```python
from build123d import *

# Parameters (mm, degrees)
BOSS_EXTRU_1_DEPTH       = 35
COQUE3_T                 = 2
ESQUISSE3_R              = 13
ENL_V_MAT_EXTRU_1_DEPTH  = 82.443231763
ESQUISSE5_W              = 20
ESQUISSE5_H              = 5
ENL_V_MAT_EXTRU_3_DEPTH  = 2
ESQUISSE6_R              = 4.6
ENL_V_MAT_EXTRU_4_DEPTH  = 122.428991596
ESQUISSE7_R              = 2.1
ENL_V_MAT_EXTRU_5_DEPTH  = 122.428991596
ESQUISSE8_W              = 44
ESQUISSE8_H              = 20
BOSS_EXTRU_2_DEPTH       = 17
ESQUISSE9_W              = 40
ESQUISSE9_H              = 15
ENL_V_MAT_EXTRU_7_DEPTH  = 18
ESQUISSE10_W             = 3
ESQUISSE10_H             = 6
ENL_V_MAT_EXTRU_8_DEPTH  = 5
BOSS_EXTRU_4_DEPTH       = 3
ESQUISSE22_R             = 4.5
BOSS_EXTRU_7_DEPTH       = 1
ENL_V_START              = -3
ESQUISSE24_R             = 2.1
ENL_V_MAT_EXTRU_12_DEPTH = 3
ESQUISSE20_R             = 4.5
BOSS_EXTRU_8_DEPTH       = 1
ESQUISSE25_R             = 2.1
ENL_V_MAT_EXTRU_13_DEPTH = 3
BOSS_EXTRU_9_START       = 1
ESQUISSE26_R             = 4.5
BOSS_EXTRU_9_DEPTH       = 1
ESQUISSE27_R             = 2.1
ENL_V_MAT_EXTRU_14_DEPTH = 3
BOSS_EXTRU_10_START      = 1
ESQUISSE28_R             = 4.5
BOSS_EXTRU_10_DEPTH      = 1
ESQUISSE29_R             = 2.1
ENL_V_MAT_EXTRU_15_DEPTH = 3
ESQUISSE34_R             = 5.75
BOSS_EXTRU_16_DEPTH      = 1
ESQUISSE35_R             = 4.6
ENL_V_MAT_EXTRU_19_DEPTH = 1
ESQUISSE36_R             = 5.5
BOSS_EXTRU_17_DEPTH      = 1
ESQUISSE37_R             = 4.6
ENL_V_MAT_EXTRU_20_DEPTH = 1
NERVURE3_REACH           = 96.86
ESQUISSE38_WALL_W        = 204.379203954
ESQUISSE38_WALL_H        = 2
NERVURE4_REACH           = 120.87
ESQUISSE39_WALLS_W       = 252.639353074
ESQUISSE39_WALLS_H       = 2
ESQUISSE40_W             = 24
ESQUISSE40_H             = 20
ENL_V_MAT_EXTRU_21_DEPTH = 2
SYM_TRIE2_START          = 12.2
SYM_TRIE2_OUTLINE_W      = 1
SYM_TRIE2_OUTLINE_H      = 11.067979308
SYM_TRIE2_DEPTH          = 2


with BuildPart() as part:
    # Esquisse1 → Boss.-Extru.1 (new body)
    with BuildSketch(Plane.XY):
        Polygon((-50, 20), (-20, 50), (20, 50), (50, 20), (50, -50), (-50, -50), align=None)
    extrude(amount=BOSS_EXTRU_1_DEPTH)

    # Coque3
    coque3_openings = [part.faces().sort_by_distance(p)[0] for p in [
        (0, -3.956043956, 35),
    ]]
    offset(amount=COQUE3_T, openings=coque3_openings, kind=Kind.INTERSECTION)

    # Esquisse3 → Enlèv. mat.-Extru.1 (cut, through all)
    with BuildSketch(Plane.XY):
        Circle(ESQUISSE3_R)
    extrude(amount=-ENL_V_MAT_EXTRU_1_DEPTH, mode=Mode.SUBTRACT)

    # Esquisse5 → Enlèv. mat.-Extru.3 (cut)
    with BuildSketch(Plane.XZ.offset(52)):
        with Locations((39, 3.5)):
            Rectangle(ESQUISSE5_W, ESQUISSE5_H)
        with Locations((-39, 3.5)):
            Rectangle(ESQUISSE5_W, ESQUISSE5_H)
    extrude(amount=-ENL_V_MAT_EXTRU_3_DEPTH, mode=Mode.SUBTRACT)

    # Esquisse6 → Enlèv. mat.-Extru.4 (cut, through all)
    with BuildSketch(Plane.ZY.offset(52)):
        with Locations(Location((6, -3.111572875, 0), (0, 0, 270))):
            Circle(ESQUISSE6_R)
    extrude(amount=-ENL_V_MAT_EXTRU_4_DEPTH, mode=Mode.SUBTRACT)

    # Esquisse7 → Enlèv. mat.-Extru.5 (cut, through all)
    with BuildSketch(Plane.ZY.offset(52)):
        with Locations(Location((15, 14.388427125, 0), (0, 0, 270))):
            Circle(ESQUISSE7_R)
        with Locations(Location((15, -19.2, 0), (0, 0, 270))):
            Circle(ESQUISSE7_R)
    extrude(amount=-ENL_V_MAT_EXTRU_5_DEPTH, mode=Mode.SUBTRACT)

    # Esquisse8 → Boss.-Extru.2 (add)
    with BuildSketch(Plane(origin=(0, -50, 0), x_dir=(1, 0, 0), z_dir=(0, 1, 0))):
        with Locations((0, -12.381067223)):
            Rectangle(ESQUISSE8_W, ESQUISSE8_H)
    extrude(amount=BOSS_EXTRU_2_DEPTH)

    # Esquisse9 → Enlèv. mat.-Extru.7 (cut)
    with BuildSketch(Plane.XY.offset(22.381067223)):
        with Locations((0, -42.5)):
            Rectangle(ESQUISSE9_W, ESQUISSE9_H)
    extrude(amount=-ENL_V_MAT_EXTRU_7_DEPTH, mode=Mode.SUBTRACT)

    # Esquisse10 → Enlèv. mat.-Extru.8 (cut)
    with BuildSketch(Plane(origin=(-20, 0, 0), x_dir=(0, 0, -1), z_dir=(1, 0, 0))):
        with Locations((-5.881067223, -47)):
            Rectangle(ESQUISSE10_W, ESQUISSE10_H)
    extrude(amount=-ENL_V_MAT_EXTRU_8_DEPTH, mode=Mode.SUBTRACT)

    # Esquisse17 → Boss.-Extru.4 (add)
    with BuildSketch(Plane.XY.offset(35)):
        Polygon((50, -50), (50, 20), (20, 50), (-20, 50), (-50, 20), (-50, -50), align=None)
        Polygon((-47, -47), (47, -47), (47, 18.757359313), (18.757359313, 47), (-18.757359313, 47), (-47, 18.757359313), align=None, mode=Mode.SUBTRACT)
    extrude(amount=-BOSS_EXTRU_4_DEPTH)

    # Esquisse22 → Boss.-Extru.7 (add)
    with BuildSketch(Plane(origin=(-50, 0, 0), x_dir=(0, 0, -1), z_dir=(1, 0, 0))):
        with Locations(Location((-15, -19.2, 0), (0, 0, 90))):
            Circle(ESQUISSE22_R)
    extrude(amount=BOSS_EXTRU_7_DEPTH)

    # Esquisse24 → Enlèv. mat.-Extru.12 (cut)
    with BuildSketch(Plane(origin=(-49, 0, 0), x_dir=(0, 0, -1), z_dir=(1, 0, 0)).offset(ENL_V_START)):
        with Locations(Location((-15, -19.2, 0), (0, 0, 270))):
            Circle(ESQUISSE24_R)
    extrude(amount=ENL_V_MAT_EXTRU_12_DEPTH, mode=Mode.SUBTRACT)

    # Esquisse20 → Boss.-Extru.8 (add)
    with BuildSketch(Plane(origin=(-50, 0, 0), x_dir=(0, 0, -1), z_dir=(1, 0, 0))):
        with Locations(Location((-15, 14.388427125, 0), (0, 0, 90))):
            Circle(ESQUISSE20_R)
    extrude(amount=BOSS_EXTRU_8_DEPTH)

    # Esquisse25 → Enlèv. mat.-Extru.13 (cut)
    with BuildSketch(Plane.ZY.offset(50)):
        with Locations(Location((15, 14.388427125, 0), (0, 0, 270))):
            Circle(ESQUISSE25_R)
    extrude(amount=-ENL_V_MAT_EXTRU_13_DEPTH, mode=Mode.SUBTRACT)

    # Esquisse26 → Boss.-Extru.9 (add)
    with BuildSketch(Plane.ZY.offset(-50).offset(BOSS_EXTRU_9_START)):
        with Locations(Location((15, 14.388427125, 0), (0, 0, 90))):
            Circle(ESQUISSE26_R)
    extrude(amount=-BOSS_EXTRU_9_DEPTH)

    # Esquisse27 → Enlèv. mat.-Extru.14 (cut)
    with BuildSketch(Plane(origin=(50, 0, 0), x_dir=(0, 0, -1), z_dir=(1, 0, 0)).offset(ENL_V_START)):
        with Locations(Location((-15, 14.388427125, 0), (0, 0, 270))):
            Circle(ESQUISSE27_R)
    extrude(amount=ENL_V_MAT_EXTRU_14_DEPTH, mode=Mode.SUBTRACT)

    # Esquisse28 → Boss.-Extru.10 (add)
    with BuildSketch(Plane.ZY.offset(-50).offset(BOSS_EXTRU_10_START)):
        with Locations(Location((15, -19.2, 0), (0, 0, 90))):
            Circle(ESQUISSE28_R)
    extrude(amount=-BOSS_EXTRU_10_DEPTH)

    # Esquisse29 → Enlèv. mat.-Extru.15 (cut)
    with BuildSketch(Plane.ZY.offset(-49)):
        with Locations(Location((15, -19.2, 0), (0, 0, 270))):
            Circle(ESQUISSE29_R)
    extrude(amount=-ENL_V_MAT_EXTRU_15_DEPTH, mode=Mode.SUBTRACT)

    # Esquisse34 → Boss.-Extru.16 (add)
    with BuildSketch(Plane(origin=(-50, 0, 0), x_dir=(0, 0, -1), z_dir=(1, 0, 0))):
        with Locations(Location((-6, -3.111572875, 0), (0, 0, 90))):
            Circle(ESQUISSE34_R)
    extrude(amount=BOSS_EXTRU_16_DEPTH)

    # Esquisse35 → Enlèv. mat.-Extru.19 (cut)
    with BuildSketch(Plane.ZY.offset(50)):
        with Locations(Location((6, -3.111572875, 0), (0, 0, 270))):
            Circle(ESQUISSE35_R)
    extrude(amount=-ENL_V_MAT_EXTRU_19_DEPTH, mode=Mode.SUBTRACT)

    # Esquisse36 → Boss.-Extru.17 (add)
    with BuildSketch(Plane.ZY.offset(-50)):
        with Locations((6, -3.111572875)):
            Circle(ESQUISSE36_R)
    extrude(amount=BOSS_EXTRU_17_DEPTH)

    # Esquisse37 → Enlèv. mat.-Extru.20 (cut)
    with BuildSketch(Plane.ZY.offset(-49)):
        with Locations(Location((6, -3.111572875, 0), (0, 0, 270))):
            Circle(ESQUISSE37_R)
    extrude(amount=-ENL_V_MAT_EXTRU_20_DEPTH, mode=Mode.SUBTRACT)

    # Esquisse38 wall → Nervure3 (add, up to next)
    with BuildSketch(Plane(origin=(-48, -19.2, 25.75), x_dir=(-0.157990501107, 0, -0.987440631917), z_dir=(-0.987440631917, 0, 0.157990501107)), mode=Mode.PRIVATE) as nervure3_sk1:
        Rectangle(ESQUISSE38_WALL_W, ESQUISSE38_WALL_H)
    nervure3_tool1 = extrude(nervure3_sk1.sketch, amount=NERVURE3_REACH, mode=Mode.PRIVATE) - part.part
    nervure3 = nervure3_tool1.solids().sort_by_distance((-48, -19.2, 25.75))[0]
    add(nervure3)

    # Esquisse39 walls → Nervure4 (add, up to next)
    with BuildSketch(Plane(origin=(-49, 0, 0), x_dir=(0, 0, -1), z_dir=(1, 0, 0)), mode=Mode.PRIVATE) as nervure4_sk1:
        with Locations((-6.45, -19.2)):
            Rectangle(ESQUISSE39_WALLS_W, ESQUISSE39_WALLS_H)
    nervure4_tool1 = extrude(nervure4_sk1.sketch, amount=-NERVURE4_REACH, mode=Mode.PRIVATE) - part.part
    nervure4 = nervure4_tool1.solids().sort_by_distance((-49, -19.2, 6.45))[0]
    add(nervure4)

    # Esquisse40 → Enlèv. mat.-Extru.21 (cut)
    with BuildSketch(Plane(origin=(0, -33, 0), x_dir=(1, 0, 0), z_dir=(0, 1, 0))):
        with Locations((0, -12.381067223)):
            Rectangle(ESQUISSE40_W, ESQUISSE40_H)
    extrude(amount=-ENL_V_MAT_EXTRU_21_DEPTH, mode=Mode.SUBTRACT)

    # Symétrie1: Nervure3, Nervure4 across plane
    add(nervure3.mirror(Plane(origin=(0, 0, 0), x_dir=(0, 0, 1), z_dir=(1, 0, 0))))
    add(nervure4.mirror(Plane(origin=(0, 0, 0), x_dir=(0, 0, 1), z_dir=(1, 0, 0))))

    # Symétrie2: read off the stored shape, not the designer's step
    # Symétrie2 outline → Symétrie2 (add)
    with BuildSketch(Plane(origin=(0, 0, 0), x_dir=(1, 0, 0), z_dir=(0, 1, 0)).offset(SYM_TRIE2_START)):
        Polygon((47, -32), (50, -32), (50, -18.932020692), (49.090876689, -18.932020692), align=None)
        with Locations((49.5, -5.533989654)):
            Rectangle(SYM_TRIE2_OUTLINE_W, SYM_TRIE2_OUTLINE_H)
        Polygon((-49.090876689, -18.932020692), (-50, -18.932020692), (-50, -32), (-47, -32), align=None)
        with Locations((-49.5, -5.533989654)):
            Rectangle(SYM_TRIE2_OUTLINE_W, SYM_TRIE2_OUTLINE_H)
    extrude(amount=SYM_TRIE2_DEPTH)


solid = part.part
```
Geometry: final body of the model. Coordinates: model frame, mm. A direction names the side the tool comes from. Round coordinates to 2 decimals unless told otherwise and drop trailing zeros. Order: outer loops, then holes, each group sorted by start corner. A loop starts at its lowest first (then second) coordinate and runs counter-clockwise, first axis right, second up. Notation, with made-up numbers: (19.5, 80) -> (44.5, 80) arc R28 cw to (44.5, 99) -> close; hole circle Ø6 at (35.25, 48). An arc over 180 degrees is marked (long way). Use CSV: the item, a comma, the result in double quotes. Start each with the question number.
1) Section C-C (x = -16). Return the cut outline in (y, z).
2) Material intervals for line 1 along Y through (x, z) = (16, 15); line 2 along Z through (x, y) = (44.5, 24); line 3 along Z through (x, y) = (-51.3, -19.2), sorted ascending. Write a range as from..to.
3) Set-up query: faces 4 (the face through (49, -20.2, 27)), 5 (the face through (17, -33, 12)), 6 (the face through (-50.521, 12.385, 15.631)). Return all of +Z, -Z, +X, -X, +Y, -Y with unobstructed straight access to the full face (end or side cutting, diameter ignored); none if empty.
4) Section B-B (z = 26). Return the cut outline in (x, y), and give its area (3 significant figures).
5) Section D-D (y = 0). State how many separate pieces and enclosed holes the cut face has, and give its area (3 significant figures).
6) Draft query along Z for faces 1 (the face through (-52, -16, 16)), 2 (the face through (12, -11, -2)), 3 (the face through (48, -3, 32)). Return one class per face: +Z half, -Z half, draft (parallel to the pull), parting line (faces both ways), or undercut.
7) Section A-A (x = 0). Return the cut outline in (y, z).
8) First-contact query: pin 1 Ø5 at (x, y) = (14, -1.5) entering from +Z; pin 2 Ø6.5 at (y, z) = (14.39, 15) entering from -X; pin 3 Ø0.8 at (x, z) = (-49.5, 6.5) entering from +Y; pin 4 Ø8 at (x, z) = (41, 24.5) entering from +Y. Flat tips, straight axial feed; report the tip coordinate or a pass-through.
Returned:
1,outline,"(-52, -2) -> (52, -2) -> (52, 35) -> (47, 35) -> (47, 32) -> (50, 32) -> (50, 0) -> (-50, 0) -> (-50, 2.38) -> (-33, 2.38) -> (-33, 22.38) -> (-35, 22.38) -> (-35, 4.38) -> (-50, 4.38) -> (-50, 32) -> (-47, 32) -> (-47, 35) -> (-52, 35) -> close"
2,line 1,"y = -52..-50, -35..-33, 50..52"
2,line 2,"z = -2..0, 32..35"
2,line 3,"z = -2..12.9, 17.1..35"
3,face 4,"none"
3,face 5,"+Z"
3,face 6,"+X, -X"
4,outline,"(-52, -52) -> (52, -52) -> (52, 20.83) -> (20.83, 52) -> (-20.83, 52) -> (-52, 20.83) -> close; hole (-50, -50) -> (50, -50) -> (50, -20.2) -> (47.96, -20.2) -> (47.96, -18.2) -> (50, -18.2) -> (50, 12.2) -> (47.96, 12.2) -> (47.96, 14.2) -> (50, 14.2) -> (50, 20) -> (20, 50) -> (-20, 50) -> (-50, 20) -> (-50, 14.2) -> (-47.96, 14.2) -> (-47.96, 12.2) -> (-50, 12.2) -> (-50, -18.2) -> (-47.96, -18.2) -> (-47.96, -20.2) -> (-50, -20.2) -> close"
4,area,"761 mm²"
5,separate pieces,"4"
5,enclosed holes,"0"
5,area,"292 mm²"
6,face 1,"draft"
6,face 2,"-Z half"
6,face 3,"undercut"
7,outline,"(-52, -2) -> (-13, -2) -> (-13, 0) -> (-50, 0) -> (-50, 2.38) -> (-35, 2.38) -> (-35, 4.38) -> (-50, 4.38) -> (-50, 32) -> (-47, 32) -> (-47, 35) -> (-52, 35) -> close; (13, -2) -> (52, -2) -> (52, 35) -> (47, 35) -> (47, 32) -> (50, 32) -> (50, 0) -> (13, 0) -> close"
8,pin 1,"stops at z = 0"
8,pin 2,"stops at x = -52"
8,pin 3,"stops at y = 23.73"
8,pin 4,"stops at y = 35.83"
